Input: part model. Units: mm. Frame: model coordinates. Face numbers are marked on the shaded views. A direction names the side the tool comes from. Give positions to 0.01 mm unless a question says otherwise; leave off trailing zeros. Loops run counter-clockwise (first coordinate to the right, second up) from the corner with the lowest first, then second, coordinate; pieces in that order, holes last. Notation, with made-up numbers: (6, 26.25) - (26, 26.25) arc R6 ccw to (26, 33.25) - close; hole circle Ø11 at (2.5, 13.25). An arc over 180 degrees is marked (long way). Answer as a JSON object with one key per item and string values.
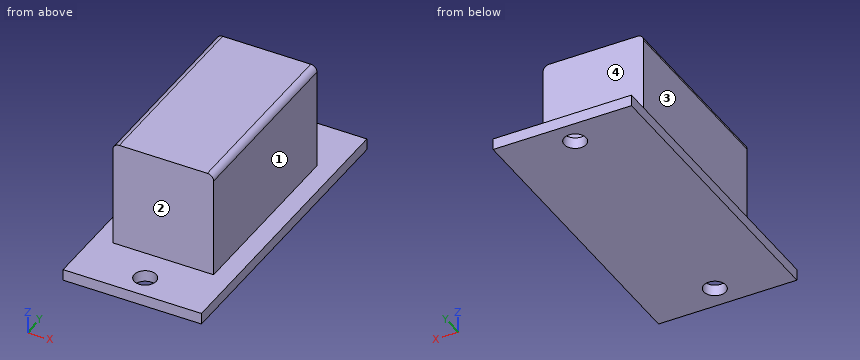
from build123d import *

# Parameters (mm, degrees)
SKETCH_1_W      = 22
SKETCH_1_H      = 48
SKETCH_1_R      = 1.75
EXTRUDE_1_DEPTH = 1.8
SKETCH_2_W      = 16
SKETCH_2_H      = 30
EXTRUDE_2_DEPTH = 17
FILLET_1_R      = 1


with BuildPart() as part:
    # 草图1 → 拉伸1 (new body)
    with BuildSketch(Plane.XY):
        Rectangle(SKETCH_1_W, SKETCH_1_H)
        with Locations((0, 20.25)):
            Circle(SKETCH_1_R, mode=Mode.SUBTRACT)
        with Locations(Location((0, -20.25, 0), (0, 0, 180))):
            Circle(SKETCH_1_R, mode=Mode.SUBTRACT)
    extrude(amount=EXTRUDE_1_DEPTH)

    # 草图2 → 拉伸2 (add)
    with BuildSketch(Plane.XY.offset(1.8)):
        Rectangle(SKETCH_2_W, SKETCH_2_H)
    extrude(amount=EXTRUDE_2_DEPTH)

    # 圆角1
    fillet_1_edges = [part.edges().sort_by_distance(p)[0] for p in [
        (-8, 0, 18.8),
        (8, 0, 18.8),
    ]]
    fillet(fillet_1_edges, radius=FILLET_1_R)


solid = part.part
Item 1: Cut plane B-B (y = -20.25). Return loops of the section in (x, z).
Geometry check:
{"outline": "(-11, 0) - (-1.75, 0) - (-1.75, 1.8) - (-11, 1.8) - close; (1.75, 0) - (11, 0) - (11, 1.8) - (1.75, 1.8) - close"}
Item 2: Access query for the marked faces 1, 2, 3 and 4. Directions: +Z, -Z, +X, -X, +Y, -Y. A direction counts if a zero-diameter tool reaches every point of the face in a straight line with its end or side. Return the directions, or none.
Geometry check:
{"face 1": "+Z, +X, +Y, -Y", "face 2": "+Z, +X, -X, -Y", "face 3": "+Z, -X, +Y, -Y", "face 4": "+Z, +X, -X, +Y"}
Item 3: Cut plane A-A (x = 0). Return loops of the section in (y, z), then the cut area to 3 significant figures.
Geometry check:
{"outline": "(-24, 0) - (-22, 0) - (-22, 1.8) - (-24, 1.8) - close; (-18.5, 0) - (18.5, 0) - (18.5, 1.8) - (15, 1.8) - (15, 18.8) - (-15, 18.8) - (-15, 1.8) - (-18.5, 1.8) - close; (22, 0) - (24, 0) - (24, 1.8) - (22, 1.8) - close", "area": "584 mm2"}
Item 4: Cut plane D-D (x = -6). Return loops of the section in (y, z), then the cut area to 3 significant figures.
Geometry check:
{"outline": "(-24, 0) - (24, 0) - (24, 1.8) - (15, 1.8) - (15, 18.8) - (-15, 18.8) - (-15, 1.8) - (-24, 1.8) - close", "area": "596 mm2"}
Item 5: Cut plane C-C (y = 11.5). Return loops of the section in (x, z).
Geometry check:
{"outline": "(-11, 0) - (11, 0) - (11, 1.8) - (8, 1.8) - (8, 17.8) arc R1 ccw to (7, 18.8) - (-7, 18.8) arc R1 ccw to (-8, 17.8) - (-8, 1.8) - (-11, 1.8) - close"}
Item 6: Contact query for flat-ended pins moving along their axis: P1, Ø10, axis at y = 16, z = 16, coming from the +X side; P2, Ø3, axis at y = 13, z = 15.5, coming from the -X side; P3, Ø4.5, axis at x = 0, y = -20.25, coming from the -Z side; P4, Ø2, axis at x = 0, y = 20.25, coming from the +Z side. Output: stop coordinate, or through.
Geometry check:
{"P1": "stops at x = 8", "P2": "stops at x = -8", "P3": "stops at z = 0", "P4": "passes through"}
Item 7: Material intervals for line 1 (Y direction, x = 0, z = 0.8); line 2 (X direction, y = -20.25, z = 0.7); line 3 (Z direction, x = -9.5, y = -8), sorted ascending. Write a range as [from, to].
Geometry check:
{"line 1": "y = [-24, -22], [-18.5, 18.5], [22, 24]", "line 2": "x = [-11, -1.75], [1.75, 11]", "line 3": "z = [0, 1.8]"}
